```python
from build123d import *

# Parameters (mm, degrees)
SKETCH_1_W             = 42
SKETCH_1_H             = 21
EXTRUDE_1_DEPTH        = 5
SKETCH_2_W             = 25
SKETCH_2_H             = 8
CUT_EXTRUDE_1_DEPTH    = 26.51960031
HOLE_WIZARD_M4_1_D     = 3.3
HOLE_WIZARD_M4_1_DEPTH = 10.1
HOLE_WIZARD_M4_1_TIP   = 0.991420021
HOLE_WIZARD_M5_1_D     = 4.2
CHAMFER_1_SIZE         = 10


with BuildPart() as part:
    # 草图1 → 凸台-拉伸1 (new, symmetric)
    with BuildSketch(Plane.XY):
        Rectangle(SKETCH_1_W, SKETCH_1_H)
    extrude(amount=EXTRUDE_1_DEPTH, both=True)

    # 草图2 → 切除-拉伸1 (cut, through all)
    with BuildSketch(Plane.XY.offset(5)):
        with Locations((0, -6.5)):
            Rectangle(SKETCH_2_W, SKETCH_2_H)
    extrude(amount=-CUT_EXTRUDE_1_DEPTH, mode=Mode.SUBTRACT)

    # M4 螺纹孔1
    with Locations(Plane(origin=(0, -10.5, 0), x_dir=(-1, 0, 0), z_dir=(0, -1, 0))):
        with Locations((16, 0), (-16, 0)):
            Hole(HOLE_WIZARD_M4_1_D / 2, depth=HOLE_WIZARD_M4_1_DEPTH)
            with Locations((0, 0, -(HOLE_WIZARD_M4_1_DEPTH + HOLE_WIZARD_M4_1_TIP / 2))):  # 118° drill point
                Cone(0, HOLE_WIZARD_M4_1_D / 2, HOLE_WIZARD_M4_1_TIP, mode=Mode.SUBTRACT)

    # M5 螺纹孔1 (through all)
    with Locations(Plane.XY.offset(5)):
        with Locations((0, 5.5)):
            Hole(HOLE_WIZARD_M5_1_D / 2)

    # 倒角1
    chamfer_1_edges = [part.edges().sort_by_distance(p)[0] for p in [
        (-21, 10.5, 0),
        (21, 10.5, 0),
    ]]
    chamfer(chamfer_1_edges, length=CHAMFER_1_SIZE)


solid = part.part
```
Part model, mm, in its own coordinate system. A direction names the side the tool comes from. Give positions to 0.01 mm unless a question says otherwise; leave off trailing zeros. Loops run counter-clockwise (first coordinate to the right, second up) from the corner with the lowest first, then second, coordinate; pieces in that order, holes last. Notation, with made-up numbers: M -36,-36.5 L -7,-36.5 A26 cw -7,0.5 Z; hole C 6.25,3.5 d9. An arc over 180 degrees is marked long. Return JSON: item names as keys, results as strings.
1) Saw through at A-A, the plane y = -7.25. List the corners of the cut face in (x, z), then the cut area to 3 significant figures.
Calculated:
{"outline": "M -21,-5 L -12.5,-5 L -12.5,5 L -21,5 Z; M 12.5,-5 L 21,-5 L 21,5 L 12.5,5 Z; hole C -16,0 d3.3; hole C 16,0 d3.3", "area": "153 mm2"}
2) Drill centre lines: line 1 (Z direction, x = 16, y = -4); line 2 (Y direction, x = 0, z = -0.5); line 3 (X direction, y = -2, z = 0.25). Where is each one in solid material? Low to high.
Calculated:
{"line 1": "z = -5 to -1.65, 1.65 to 5", "line 2": "y = -2.5 to 3.4, 7.6 to 10.5", "line 3": "x = -21 to -17.63, -14.37 to 14.37, 17.63 to 21"}
3) Pull direction X, two halves, no side cores. Call faces 4 (the face through (-14.476, -5.379, 0.632)), 5 (the face through (0, 0, 5)), 6 (the face through (21, -5, 0)): released by +X, released by -X, zero draft, split by the parting line, or undercut.
Calculated:
{"face 4": "undercut", "face 5": "zero draft", "face 6": "released by +X"}
4) Flat gauge pins, fed straight in: pin 1 Ø1.5 at (y, z) = (4.5, -1.5) entering from -X; pin 2 Ø2 at (y, z) = (5, -1.5) entering from -X; pin 3 Ø2 at (x, z) = (16, 0) entering from -Y. Where does each tip first touch, or does it go through?
Calculated:
{"pin 1": "stops at x = -17.75", "pin 2": "stops at x = -17.5", "pin 3": "stops at y = -0.01"}
5) Saw through at C-C, the plane x = 0. List the corners of the cut face in (y, z), then the cut area to 3 significant figures.
Calculated:
{"outline": "M -2.5,-5 L 3.4,-5 L 3.4,5 L -2.5,5 Z; M 7.6,-5 L 10.5,-5 L 10.5,5 L 7.6,5 Z", "area": "88.0 mm2"}
6) Saw through at D-D, the plane y = 6.5. List the corners of the cut face in (x, z).
Calculated:
{"outline": "M -15,-5 L -1.85,-5 L -1.85,5 L -15,5 Z; M 1.85,-5 L 15,-5 L 15,5 L 1.85,5 Z"}
7) 3-axis set-ups, long thin cutter, end or side, ignore diameter. For faces 1 (the face through (0, -2.5, 0)), 2 (the face through (0, 10.5, 0)), 3 (the face through (17.574, -5.379, -0.496)): which of +Z, -Z, +X, -X, +Y, -Y reach the whole face in a straight line?
Calculated:
{"face 1": "+Z, -Z, -Y", "face 2": "+Z, -Z, +X, -X, +Y", "face 3": "-Y"}
8) Saw through at B-B, the plane z = 4. List the corners of the cut face in (x, y).
Calculated:
{"outline": "M -21,-10.5 L -12.5,-10.5 L -12.5,-2.5 L 12.5,-2.5 L 12.5,-10.5 L 21,-10.5 L 21,0.5 L 11,10.5 L -11,10.5 L -21,0.5 Z; hole C 0,5.5 d4.2"}
